Check sheet for the modelled part. Datum: model origin and axes. Units: mm. A direction names the side the tool comes from. Give positions to 0.01 mm unless a question says otherwise; leave off trailing zeros. Write each loop counter-clockwise with the first axis right and the second up, starting at its lowest first coordinate (ties: lowest second). Pieces come first, ordered by that corner, then holes. Notation, with made-up numbers: M 69.5,82 L 113.5,82 A24 ccw 113.5,103 Z; hole C -28,-33 d8. An arc over 180 degrees is marked long. Write item = value, one per line. Start each with the question number.
1) Cross-section at C-C, the plane y = -18.5. Record the cut outline in (x, z), plus the area to 3 significant figures.
2) Access from +Z, -Z, +X, -X, +Y, -Y to the whole of each face (thin tool, end or side, straight path). Record for faces 4 (the cylindrical face through (130.197, 37.922, -54.289)), 5 (the flat face through (251, -12.7, 34)), 6 (the flat face through (85, 50.8, -43)), 7 (the cylindrical face through (-54.635, -0.178, 21.756)), 8 (the flat face through (87, -7, -83.939)).
3) Cross-section at A-A, the plane x = 20. Record the cut outline in (y, z), plus the area to 3 significant figures.
4) Go/stop test with flat-tipped pins: pin 1 (10 mm diameter, centred on y = 16.5, z = -56.5, fed in from -X); pin 2 (8 mm diameter, centred on y = 2.5, z = -108.5, fed in from +X); pin 3 (8 mm diameter, centred on x = -20.5, y = 14.5, fed in from -Z). Record where each tip stops, or that it passes through.
5) Cross-section at D-D, the plane x = 261. Record the cut outline in (y, z), plus the area to 3 significant figures.
6) Scan lines: line 1 along Y through (x, z) = (0, -137); line 2 along X through (y, z) = (20, -14); line 3 along Y through (x, z) = (157, 2). Record each from-to range of solid material in increasing order. Write a range as [from, to].
7) Cross-section at B-B, the plane z = 48. Give the number of separate pieces and of enclosed holes in the cut face, plus the area to 3 significant figures.
8) Mould release check, pull along Z, two halves, no side actions. Record for faces 1 (the cylindrical face through (47.537, 37.922, -55.137)), 2 (the flat face through (87, -38.1, -88)), 3 (the cylindrical face through (145.34, 0.18, -97.13)): released by +Z, released by -Z, zero draft, split by the parting line, or undercut.
```python
from build123d import *

# Parameters (mm, degrees)
F1_DEPTH  = 50.8
F3_DEPTH  = 76.2
F4_R      = 38.1
F1_FACE_R = 12.7
F5_DEPTH  = 12.7
F6_R      = 9.525
F7_DEPTH  = 25.401


with BuildPart() as f1:
    # F0 (on Front) → F1 (new body, symmetric)
    with BuildSketch(Plane.XZ):
        with BuildLine():
            ThreePointArc((-81.1352841451, 30.047498821), (-98.4838067731, 47.3960214491), (-74.7852841451, 41.0460214491))
            Line((-74.7852841451, 41.0460214491), (-55.7352841451, 41.0460214491))
            ThreePointArc((-55.7352841451, 41.0460214491), (-114.9815907152, 56.9210214491), (-71.6102841451, 13.5497148789))
            Line((-71.6102841451, 13.5497148789), (-81.1352841451, 30.047498821))
        make_face()
        with BuildLine():
            ThreePointArc((294.63812316, 41.0460214491), (262.88812316, 72.7960214491), (231.13812316, 41.0460214491))
            Line((231.13812316, 41.0460214491), (250.18812316, 41.0460214491))
            ThreePointArc((250.18812316, 41.0460214491), (262.88812316, 53.7460214491), (275.58812316, 41.0460214491))
            ThreePointArc((275.58812316, 41.0460214491), (269.23812316, 30.047498821), (256.53812316, 30.047498821))
            Line((256.53812316, 30.047498821), (247.01312316, 13.5497148789))
            ThreePointArc((247.01312316, 13.5497148789), (278.76312316, 13.5497148789), (294.63812316, 41.0460214491))
        make_face()
        with BuildLine():
            ThreePointArc((195.6514195075, -130.4039785509), (191.3977260776, -114.5289785509), (179.7764195075, -102.9076719808))
            Line((179.7764195075, -102.9076719808), (170.2514195075, -119.4054559229))
            ThreePointArc((170.2514195075, -119.4054559229), (174.8999421355, -124.0539785509), (176.6014195075, -130.4039785509))
            ThreePointArc((176.6014195075, -130.4039785509), (163.9014195075, -143.1039785509), (151.2014195075, -130.4039785509))
            Line((151.2014195075, -130.4039785509), (132.1514195075, -130.4039785509))
            ThreePointArc((132.1514195075, -130.4039785509), (163.9014195075, -162.1539785509), (195.6514195075, -130.4039785509))
        make_face()
        with BuildLine():
            Line((5.1514195075, -119.4054559229), (-4.3735804925, -102.9076719808))
            ThreePointArc((-4.3735804925, -102.9076719808), (-4.3735804925, -157.9002851211), (43.2514195075, -130.4039785509))
            Line((43.2514195075, -130.4039785509), (24.2014195075, -130.4039785509))
            ThreePointArc((24.2014195075, -130.4039785509), (5.1514195075, -141.402501179), (5.1514195075, -119.4054559229))
        make_face()
        with BuildLine():
            ThreePointArc((43.2514195075, -130.4039785509), (27.3764195075, -102.9076719808), (-4.3735804925, -102.9076719808))
            Line((-4.3735804925, -102.9076719808), (5.1514195075, -119.4054559229))
            ThreePointArc((5.1514195075, -119.4054559229), (17.8514195075, -119.4054559229), (24.2014195075, -130.4039785509))
            Line((24.2014195075, -130.4039785509), (43.2514195075, -130.4039785509))
        make_face()
        with BuildLine():
            Line((-55.7352841451, 41.0460214491), (-74.7852841451, 41.0460214491))
            ThreePointArc((-74.7852841451, 41.0460214491), (-76.486761517, 34.6960214491), (-81.1352841451, 30.047498821))
            Line((-81.1352841451, 30.047498821), (-71.6102841451, 13.5497148789))
            ThreePointArc((-71.6102841451, 13.5497148789), (-59.9889775749, 25.1710214491), (-55.7352841451, 41.0460214491))
        make_face()
        with BuildLine():
            Line((250.18812316, 41.0460214491), (231.13812316, 41.0460214491))
            ThreePointArc((231.13812316, 41.0460214491), (235.3918165899, 25.1710214491), (247.01312316, 13.5497148789))
            Line((247.01312316, 13.5497148789), (256.53812316, 30.047498821))
            ThreePointArc((256.53812316, 30.047498821), (251.889600532, 34.6960214491), (250.18812316, 41.0460214491))
        make_face()
        with BuildLine():
            Line((170.2514195075, -119.4054559229), (179.7764195075, -102.9076719808))
            ThreePointArc((179.7764195075, -102.9076719808), (148.0264195075, -102.9076719808), (132.1514195075, -130.4039785509))
            Line((132.1514195075, -130.4039785509), (151.2014195075, -130.4039785509))
            ThreePointArc((151.2014195075, -130.4039785509), (157.5514195075, -119.4054559229), (170.2514195075, -119.4054559229))
        make_face()
        with BuildLine():
            Line((231.13812316, 41.0460214491), (-55.7352841451, 41.0460214491))
            ThreePointArc((-55.7352841451, 41.0460214491), (-59.9889775749, 25.1710214491), (-71.6102841451, 13.5497148789))
            Line((-71.6102841451, 13.5497148789), (-4.3735804925, -102.9076719808))
            ThreePointArc((-4.3735804925, -102.9076719808), (27.3764195075, -102.9076719808), (43.2514195075, -130.4039785509))
            Line((43.2514195075, -130.4039785509), (132.1514195075, -130.4039785509))
            ThreePointArc((132.1514195075, -130.4039785509), (148.0264195075, -102.9076719808), (179.7764195075, -102.9076719808))
            Line((179.7764195075, -102.9076719808), (247.01312316, 13.5497148789))
            ThreePointArc((247.01312316, 13.5497148789), (235.3918165899, 25.1710214491), (231.13812316, 41.0460214491))
        make_face()
    extrude(amount=F1_DEPTH, both=True)

    # F2 (on face) → F3 (cut)
    with BuildSketch(Plane.XZ.offset(50.8)):
        Polygon((211.5616842291, 41.0460214491), (-36.1588452141, 41.0460214491), (36.0010718467, -83.9386211703), (139.4017671682, -83.9386211703), align=None)
    extrude(amount=-F3_DEPTH, mode=Mode.SUBTRACT)

    # F4 (on Front) + F1_face (on face) → F5 (cut, symmetric)
    with BuildSketch(Plane.XZ):
        with Locations((-87.4930471182, 41.0424880683)):
            Circle(F4_R)
        with Locations((262.2837722301, 41.0460214491)):
            Circle(F4_R)
        with Locations((163.9014195075, -130.4039785509)):
            Circle(F4_R)
        with Locations((11.5014195075, -130.4039785509)):
            Circle(F4_R)
    with BuildSketch(Plane(origin=(87.7014195075, -50.8, -33.7225685026), x_dir=(1, 0, 0), z_dir=(0, -1, 0))):
        with BuildLine():
            Line((-123.8602647216, 74.7685899517), (-143.4367036526, 74.7685899517))
            ThreePointArc((-143.4367036526, 74.7685899517), (-202.6830102227, 90.6435899517), (-159.3117036526, 47.2722833815))
            Line((-159.3117036526, 47.2722833815), (-92.075, -69.1851034782))
            ThreePointArc((-92.075, -69.1851034782), (-92.075, -124.1777166185), (-44.45, -96.6814100483))
            Line((-44.45, -96.6814100483), (44.45, -96.6814100483))
            ThreePointArc((44.45, -96.6814100483), (92.075, -124.1777166185), (92.075, -69.1851034782))
            Line((92.075, -69.1851034782), (159.3117036526, 47.2722833815))
            ThreePointArc((159.3117036526, 47.2722833815), (202.6830102227, 90.6435899517), (143.4367036526, 74.7685899517))
            Line((143.4367036526, 74.7685899517), (123.8602647216, 74.7685899517))
            Line((123.8602647216, 74.7685899517), (51.7003476608, -50.2160526677))
            Line((51.7003476608, -50.2160526677), (-51.7003476608, -50.2160526677))
            Line((-51.7003476608, -50.2160526677), (-123.8602647216, 74.7685899517))
        make_face()
        with Locations((-76.2, -96.6814100483)):
            Circle(F1_FACE_R, mode=Mode.SUBTRACT)
        with Locations((76.2, -96.6814100483)):
            Circle(F1_FACE_R, mode=Mode.SUBTRACT)
        with Locations((-175.1867036526, 74.7685899517)):
            Circle(F1_FACE_R, mode=Mode.SUBTRACT)
        with Locations((175.1867036526, 74.7685899517)):
            Circle(F1_FACE_R, mode=Mode.SUBTRACT)
    extrude(amount=F5_DEPTH, both=True, mode=Mode.SUBTRACT)

    # F6 (on face) → F7 (cut, through all)
    with BuildSketch(Plane.XZ.offset(-25.4)):
        with Locations((49.6014195075, -45.8386211703)):
            Circle(F6_R)
        with Locations((125.8014195075, -45.8386211703)):
            Circle(F6_R)
    extrude(amount=-F7_DEPTH, mode=Mode.SUBTRACT)


solid = f1.part
```
Reply:
q1.outline = M -71.61,13.55 L -4.37,-102.91 A31.75 ccw long 43.25,-130.4 L 132.15,-130.4 A31.75 ccw long 179.78,-102.91 L 247.01,13.55 A31.75 ccw long 231.14,41.05 L 211.56,41.05 L 139.4,-83.94 L 36,-83.94 L -36.16,41.05 L -55.74,41.05 A31.75 ccw long Z; hole C -87.49,41.05 d25.4; hole C 11.5,-130.4 d25.4; hole C 163.9,-130.4 d25.4; hole C 262.89,41.05 d25.4
q1.area = 28,600 mm2
q2.face_4 = +Y, -Y
q2.face_5 = +Z, +X
q2.face_6 = +Z, -Z, +X, -X, +Y
q2.face_7 = +Z, -X
q2.face_8 = +Z, -Y
q3.outline = M -38.1,-161 L -12.7,-161 L -12.7,-139.84 L -38.1,-139.84 Z; M -38.1,-120.97 L -12.7,-120.97 L -12.7,-93.26 L 12.7,-93.26 L 12.7,-120.97 L 50.8,-120.97 L 50.8,41.05 L 25.4,41.05 L 25.4,-56.22 L -38.1,-56.22 Z; M 12.7,-161 L 50.8,-161 L 50.8,-139.84 L 12.7,-139.84 Z
q3.area = 8,870 mm2
q4.pin_1 = -34.05
q4.pin_2 = 135.96
q4.pin_3 = -145.37
q5.outline = M -38.1,9.35 L -12.7,9.35 L -12.7,28.49 L -38.1,28.49 Z; M -38.1,53.6 L -12.7,53.6 L -12.7,72.74 L -38.1,72.74 Z; M 12.7,9.35 L 50.8,9.35 L 50.8,28.49 L 12.7,28.49 Z; M 12.7,53.6 L 50.8,53.6 L 50.8,72.74 L 12.7,72.74 Z
q5.area = 2,430 mm2
q6.line_1 = [-38.1, -12.7], [12.7, 50.8]
q6.line_2 = [-55.7, -4.38], [179.78, 231.11]
q6.line_3 = [25.4, 50.8]
q7.separate_pieces = 8
q7.enclosed_holes = 0
q7.area = 5,170 mm2
q8.face_1 = undercut
q8.face_2 = zero draft
q8.face_3 = released by -Z
